Model file for the job. Use its own axes, mm. A direction names the side the tool comes from. Give positions to 0.01 mm unless a question says otherwise; leave off trailing zeros. Loops run counter-clockwise (first coordinate to the right, second up) from the corner with the lowest first, then second, coordinate; pieces in that order, holes last. Notation, with made-up numbers: (-23, 52.5) - (-19, 52.5) arc R24 cw to (-19, 64.5) - close; hole circle Ø8 at (25.25, -1.5). An arc over 180 degrees is marked (long way). Use a Markdown table: item, result.
from build123d import *


with BuildPart() as part:
    # Sketch1 → Loft l2 section 0
    with BuildSketch(Plane(origin=(0, 0, 0), x_dir=(0, 0, -1), z_dir=(1, 0, 0))):
        Polygon((-231, 490), (221, 490), (221, 480), (0, 480), (0, -480), (221, -480), (221, -490), (-231, -490), (-231, -480), (-10, -480), (-10, 480), (-231, 480), align=None)
    # Sketch4 → Loft l2 section 1
    with BuildSketch(Plane(origin=(1000, 0, -1000), x_dir=(0, 0, 1), z_dir=(-1, 0, 0))):
        Polygon((881, 490), (1129, 490), (1129, 480), (1010, 480), (1010, -480), (1129, -480), (1129, -490), (881, -490), (881, -480), (1000, -480), (1000, 480), (881, 480), align=None)
    loft()


solid = part.part
(1) 3-axis set-ups, long thin cutter, end or side, ignore diameter. For faces 1 (the flat face through (507, -485.07, 179.286)), 2 (the flat face through (507, 7, 0)): which of +Z, -Z, +X, -X, +Y, -Y reach the whole face in a straight line?
Computed:
| item | result |
|---|---|
| face 1 | +Z, +X, +Y, -Y |
| face 2 | -Z, +X, -X |
(2) Slice it at A-A, the plane y = -175. Write the cut outline in (x, z).
Computed:
| item | result |
|---|---|
| outline | (0, 0) - (1000, 0) - (1000, 10) - (0, 10) - close |
(3) Mould opens along Y. For faces 3 (the flat face through (507, -7, 10)), 4 (the flat face through (0, 3, 4)) say: pulls with the +Y half, pulls with the -Y half, needs draft (parallel to the pull), parting line crosses it, or undercut.
Computed:
| item | result |
|---|---|
| face 3 | undercut |
| face 4 | needs draft |
(4) Pin check, flat tips, straight feed: P1, Ø2, axis at x = 494, y = 359, coming from the -Z side; P2, Ø4, axis at x = 742, y = 244, coming from the +Z side. Stop position of each tip, or through.
Computed:
| item | result |
|---|---|
| P1 | z = 0 |
| P2 | z = 10 |
(5) Drill centre lines: probe 1 along Y at (x, z) = (268, -107); probe 2 along Z at (x, y) = (911, 35). Where is each one in solid material? Low to high. Write a range as [from, to].
Computed:
| item | result |
|---|---|
| probe 1 | [-490, -480], [480, 490] |
| probe 2 | [0, 10] |
